Part model, mm, in its own coordinate system. A direction names the side the tool comes from. Give positions to 0.01 mm unless a question says otherwise; leave off trailing zeros. Loops run counter-clockwise (first coordinate to the right, second up) from the corner with the lowest first, then second, coordinate; pieces in that order, holes last. Notation, with made-up numbers: M 72.5,-16 L 104.5,-16 A14 cw 104.5,-11 Z; hole C -26,17.5 d7. An arc over 180 degrees is marked long. Answer in a Markdown table with one row per item.
from build123d import *

# Parameters (mm, degrees)
SKETCH2_W           = 90
SKETCH2_H           = 5
BOSS_EXTRUDE1_DEPTH = 21
SKETCH3_W           = 90
SKETCH3_H           = 5
BOSS_EXTRUDE2_DEPTH = 105
FILLET1_R           = 10
SKETCH4_R           = 4.025
CUT_EXTRUDE1_DEPTH  = 118.631840928
CUT_EXTRUDE2_DEPTH  = 119.415581745
SKETCH7_R           = 1.45
CUT_EXTRUDE4_DEPTH  = 5
SKETCH6_W           = 5.5
SKETCH6_H           = 5
SKETCH6_W_2         = 20.5
SKETCH6_H_2         = 40.9
CUT_EXTRUDE3_DEPTH  = 118.631840928
CUT_EXTRUDE5_DEPTH  = 10


with BuildPart() as part:
    # Sketch2 → Boss-Extrude1 (new body)
    with BuildSketch(Plane.XY):
        Rectangle(SKETCH2_W, SKETCH2_H)
    extrude(amount=BOSS_EXTRUDE1_DEPTH)

    # Sketch3 → Boss-Extrude2 (add)
    with BuildSketch(Plane(origin=(0, 2.5, 0), x_dir=(1, 0, 0), z_dir=(0, 1, 0))):
        with Locations((0, -2.5)):
            Rectangle(SKETCH3_W, SKETCH3_H)
    extrude(amount=BOSS_EXTRUDE2_DEPTH)

    # Fillet1
    fillet1_edges = [part.edges().sort_by_distance(p)[0] for p in [
        (-45, 107.5, 2.5),
    ]]
    fillet(fillet1_edges, radius=FILLET1_R)

    # Sketch4 → Cut-Extrude1 (cut, through all)
    with BuildSketch(Plane.XY.offset(5)):
        with Locations((-33, 95.5)):
            Circle(SKETCH4_R)
    extrude(amount=-CUT_EXTRUDE1_DEPTH, mode=Mode.SUBTRACT)

    # Sketch5 → Cut-Extrude2 (cut, through all)
    with BuildSketch(Plane.XY.offset(21)):
        Polygon((-45, 77.5), (-15, -2.5), (-45, -2.5), align=None)
        Polygon((15, 107.5), (45, 27.5), (45, 107.5), align=None)
    extrude(amount=-CUT_EXTRUDE2_DEPTH, mode=Mode.SUBTRACT)

    # Sketch7 → Cut-Extrude4 (cut)
    with BuildSketch(Plane.XY.offset(5)):
        with Locations((-13.25, 48.85)):
            Circle(SKETCH7_R)
        with Locations((-3.25, 48.85)):
            Circle(SKETCH7_R)
        with Locations((-3.25, 99.25)):
            Circle(SKETCH7_R)
        with Locations((-13.25, 99.25)):
            Circle(SKETCH7_R)
    extrude(amount=-CUT_EXTRUDE4_DEPTH, mode=Mode.SUBTRACT)

    # Sketch6 → Cut-Extrude3 (cut, through all)
    with BuildSketch(Plane.XY.offset(5)):
        with Locations((-8.25, 97)):
            Rectangle(SKETCH6_W, SKETCH6_H)
        with Locations((-8.25, 74.05)):
            Rectangle(SKETCH6_W_2, SKETCH6_H_2)
    extrude(amount=-CUT_EXTRUDE3_DEPTH, mode=Mode.SUBTRACT)

    # Sketch8 → Cut-Extrude5 (cut)
    with BuildSketch(Plane(origin=(0, 2.5, 0), x_dir=(1, 0, 0), z_dir=(0, 1, 0))):
        with BuildLine():
            Line((-6.875, -12.15), (35, -12.15))
            ThreePointArc((35, -12.15), (36.6, -13.75), (35, -15.35))
            Line((35, -15.35), (-6.875, -15.35))
            ThreePointArc((-6.875, -15.35), (-8.475, -13.75), (-6.875, -12.15))
        make_face()
    extrude(amount=-CUT_EXTRUDE5_DEPTH, mode=Mode.SUBTRACT)


solid = part.part
(1) Pull direction Z, two halves, no side cores. Call faces 4 (the face through (14, 0, 15.35)), 5 (the face through (14, 0, 21)), 6 (the face through (-10, 107.5, 2)): +Z half, -Z half, draft (parallel to the pull), parting line (faces both ways), or undercut.
Recorded:
| item | result |
|---|---|
| face 4 | undercut |
| face 5 | +Z half |
| face 6 | draft |
(2) Pin check, flat tips, straight feed: pin 1 Ø4.5 at (x, y) = (-13.25, 99.25) entering from +Z; pin 2 Ø2.5 at (y, z) = (97.5, 3) entering from +X; pin 3 Ø2.5 at (y, z) = (79.5, 1.5) entering from +X. Stop position of each tip, or through.
Recorded:
| item | result |
|---|---|
| pin 1 | stops at z = 5 |
| pin 2 | stops at x = 19.22 |
| pin 3 | stops at x = 25.97 |
(3) Which spindle directions (+Z, -Z, +X, -X, +Y, -Y) get a long thin tool onto all of the face, cutting with end or side? Do faces 1 (the face through (15, -2.5, 10)), 2 (the face through (-8, 53.6, 3)), 3 (the face through (-8.475, 0.035, 13.785)). Say none if no direction does.
Recorded:
| item | result |
|---|---|
| face 1 | +Z, -Z, +X, -X, -Y |
| face 2 | +Z, -Z |
| face 3 | +Y, -Y |
(4) Saw through at B-B (z = 1.75). Write the cut outline in (x, y) (3 decimals), plus the area to 3 significant figures.
Recorded:
| item | result |
|---|---|
| outline | M -45,77.5 L -15,-2.5 L 45,-2.5 L 45,27.5 L 15,107.5 L -35,107.5 A10 ccw -45,97.5 Z; hole C -33,95.5 d8.05; hole M -18.5,53.6 L 2,53.6 L 2,94.5 L -5.5,94.5 L -5.5,99.5 L -11,99.5 L -11,94.5 L -18.5,94.5 Z; hole C -13.25,48.85 d2.9; hole C -13.25,99.25 d2.9; hole C -3.25,48.85 d2.9; hole C -3.25,99.25 d2.9 |
| area | 6,540 mm^2 |
(5) Saw through at D-D (x = -13.25). Write the cut outline in (y, z), plus the area to 4 significant figures.
Recorded:
| item | result |
|---|---|
| outline | M -2.5,0 L 47.4,0 L 47.4,5 L 2.5,5 L 2.5,21 L -2.5,21 Z; M 50.3,0 L 53.6,0 L 53.6,5 L 50.3,5 Z; M 94.5,0 L 97.8,0 L 97.8,5 L 94.5,5 Z; M 100.7,0 L 107.5,0 L 107.5,5 L 100.7,5 Z |
| area | 396.5 mm^2 |
(6) Saw through at C-C (z = 13.75). Write the cut outline in (x, y) (3 decimals).
Recorded:
| item | result |
|---|---|
| outline | M -16.875,2.5 L -15,-2.5 L -8.475,-2.5 L -8.475,2.5 Z; M 36.6,-2.5 L 45,-2.5 L 45,2.5 L 36.6,2.5 Z |
(7) Drill centre lines: line 1 along Y through (x, z) = (-13.25, 3.2); line 2 along Y through (x, z) = (25, 6.5); line 3 along Z through (x, y) = (-24.5, 41.5). Where is each one in solid material? Low to high.
Recorded:
| item | result |
|---|---|
| line 1 | y = -2.5 to 47.4, 50.3 to 53.6, 94.5 to 97.8, 100.7 to 107.5 |
| line 2 | y = -2.5 to 2.5 |
| line 3 | z = 0 to 5 |
(8) Saw through at A-A (x = -33). Write the cut outline in (y, z) (3 decimals).
Recorded:
| item | result |
|---|---|
| outline | M 45.5,0 L 91.475,0 L 91.475,5 L 45.5,5 Z; M 99.525,0 L 107.5,0 L 107.5,5 L 99.525,5 Z |
